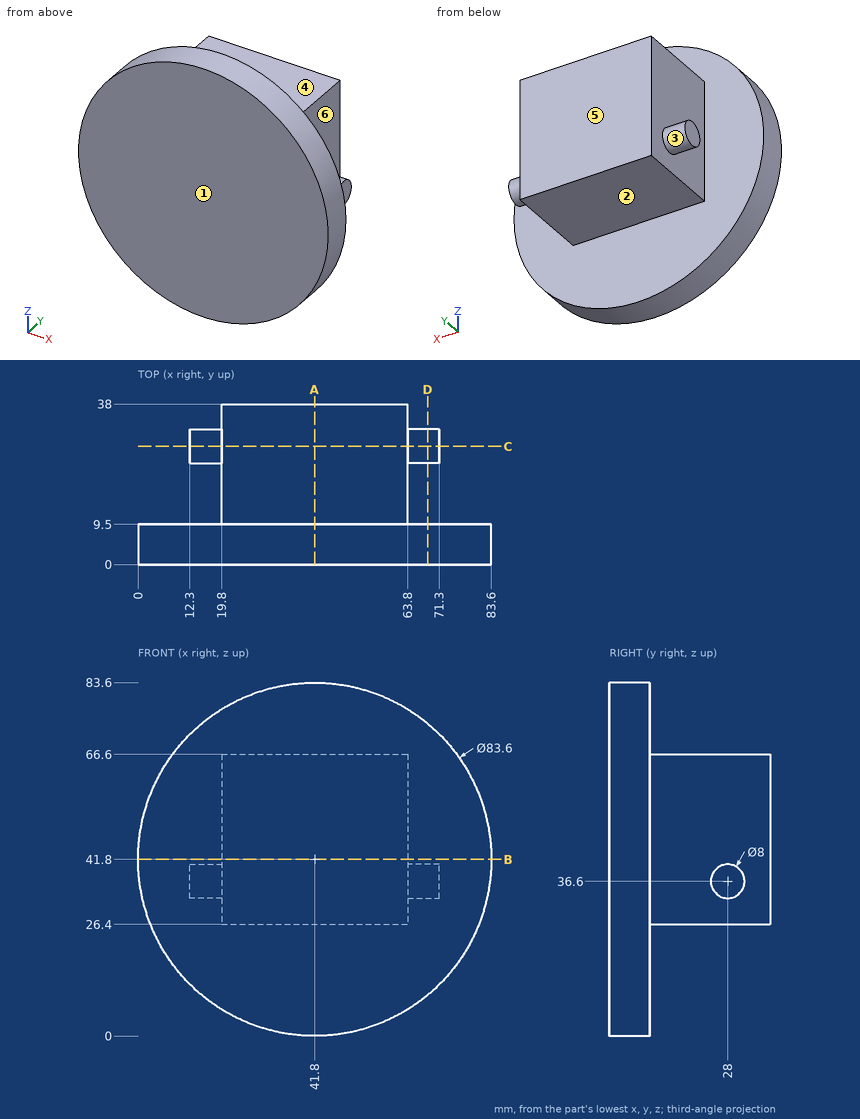
Check sheet for the drawn part. Datum: minimum x, y, z corner. Units: mm. A direction names the side the tool comes from. Give positions to 0.01 mm unless a question says otherwise; leave off trailing zeros. Loops run counter-clockwise (first coordinate to the right, second up) from the corner with the lowest first, then second, coordinate; pieces in that order, holes last. Notation, with made-up numbers: M 14.25,-11 L 19.25,-11 A17 cw 19.25,-3 Z; hole C 3.5,61 d1. An arc over 180 degrees is marked long. Answer as CSV lines item,"result".
Item 1: Draft check along Y on the marked faces 4, 5 and 6. Enter one of: pulls with the +Y half, pulls with the -Y half, needs draft (parallel to the pull), parting line crosses it, or undercut.
Reply:
face 4,"needs draft"
face 5,"pulls with the +Y half"
face 6,"undercut"
Item 2: Sectioned sample at A-A, the plane x = 41.8. Enter the section's corners in (y, z).
Reply:
outline,"M 0,0 L 9.5,0 L 9.5,26.4 L 38,26.4 L 38,66.6 L 9.5,66.6 L 9.5,83.6 L 0,83.6 Z"
Item 3: Set-up check for the marked faces 1, 2 and 3: record each of +Z, -Z, +X, -X, +Y, -Y from which the full face is reachable in a straight line by a thin tool's end or side.
Reply:
face 1,"+Z, -Z, +X, -X, -Y"
face 2,"-Z, +X, -X, +Y"
face 3,"-X"
Item 4: Scan lines: L1, parallel to Z at x = 62.5, y = 10; L2, parallel to X at y = 20.5, z = 43.5; L3, parallel to Y at x = 76.5, z = 44. Record each from-to range of solid material in increasing order.
Reply:
L1,"26.4 to 66.6"
L2,"19.8 to 63.8"
L3,"0 to 9.5"
Item 5: Sectioned sample at B-B, the plane z = 41.8. Enter the section's corners in (x, y), then the cut area to 3 significant figures.
Reply:
outline,"M 0,0 L 83.6,0 L 83.6,9.5 L 63.8,9.5 L 63.8,38 L 19.8,38 L 19.8,9.5 L 0,9.5 Z"
area,"2,050 mm^2"
Item 6: Sectioned sample at C-C, the plane y = 28. Enter the section's corners in (x, z).
Reply:
outline,"M 12.3,32.6 L 19.8,32.6 L 19.8,26.4 L 63.8,26.4 L 63.8,32.6 L 71.3,32.6 L 71.3,40.6 L 63.8,40.6 L 63.8,66.6 L 19.8,66.6 L 19.8,40.6 L 12.3,40.6 Z"
Item 7: Sectioned sample at D-D, the plane x = 68.5. Enter the section's corners in (y, z), then the cut area to 3 significant figures.
Reply:
outline,"M 0,9.64 L 9.5,9.64 L 9.5,73.96 L 0,73.96 Z; C 28,36.6 d8"
area,"661 mm^2"
Item 8: Depth check by flat-ended pin: pin 1 Ø4 at (y, z) = (27, 36) entering from -X; pin 2 Ø4 at (y, z) = (27.5, 37.5) entering from +X; pin 3 Ø12 at (x, y) = (35, 30.5) entering from -Z. Enter the tip coordinate at first touch or a pass-through.
Reply:
pin 1,"x = 12.3"
pin 2,"x = 71.3"
pin 3,"z = 26.4"
